Could you check a few things on this model? Use its own coordinates, in mm. A direction names the side the tool comes from. Coordinates: 2 decimals unless noted, no trailing zeros. Write each loop counter-clockwise with the first axis right and the second up, starting at its lowest first coordinate (ties: lowest second). Pieces come first, ordered by that corner, then holes. Notation, with made-up numbers: (82.25, 55) - (99.25, 55) arc R15 cw to (99.25, 66) - close; hole circle Ø6 at (26, 44.25). An arc over 180 degrees is marked (long way). Answer as a JSON object with one key per item and string values. Group by question number.
1) On a 3-axis mill with a long thin cutter (end or side, diameter ignored), from which of +Z, -Z, +X, -X, +Y, -Y can I reach the whole of each face in a straight line? I mean faces 5 (the flat face through (20.15, 0, 33)), 6 (the flat face through (-26.15, 0, 2)), 7 (the flat face through (20.15, 0, 13)), 8 (the cylindrical face through (-10.9, -0.1, 40)), 9 (the flat face through (-24, 0, 29.15)). Say none if no direction works.
2) Will these pins go through, and if not, where does the flat tip stop? pin 1 Ø2.5 at (x, y) = (23.5, 0) entering from -Z; pin 2 Ø6 at (x, y) = (1.5, 4) entering from +Z; pin 3 Ø4 at (x, z) = (-23.5, 1.5) entering from +Y; pin 4 Ø4 at (x, z) = (-21.5, 1.5) entering from -Y.
3) Please list where these lines run through material, in increasing order: line 1 along Y through (x, z) = (24.5, 28.65); line 2 along Z through (x, y) = (-7.9, 3.75); line 3 along X through (y, z) = (3.75, 31.5).
4) We'd pull the mould along Z, two halves only. Please class faces 1 (the cylindrical face through (-6.514, -0.139, 13.425)), 2 (the flat face through (-23, 2.5, 2)), 3 (the flat face through (24, 0, 26.6)), 4 (the flat face through (-24, 0, 26.6)): released by +Z, released by -Z, zero draft, split by the parting line, or undercut.
5) If we section it at C-C (x = 24.5): Write out the boundary of the cut face in (y, z), plus the area to 3 significant figures.
6) If we section it at B-B (x = -24.5): Write out the boundary of the cut face in (y, z).
7) If we section it at A-A (y = -5): Write out the boundary of the cut face in (x, z).
8) If we section it at D-D (y = 0): Write out the boundary of the cut face in (x, z), plus the area to 3 significant figures.
Autodesk Inventor part; units mm, degrees
ref_plane "YZ Plane" through (0, 0, 0) normal (1, 0, 0) x (0, 1, 0)
ref_plane "XZ Plane" through (0, 0, 0) normal (0, 1, 0) x (-1, 0, 0)
ref_plane "XY Plane" through (0, 0, 0) normal (0, 0, 1) x (1, 0, 0)
sketch "Sketch1" plane through (0, 0, 0) normal (0, 0, 1) x (1, 0, 0)
  line L0 (-28.21, 0) -> (28.21, 0)
  line L1 (0, -13.86) -> (0, 13.86)
  line L2 (-20.15, 9.9) -> (20.15, 9.9)
  line L3 (20.15, 9.9) -> (20.15, -9.9)
  line L4 (20.15, -9.9) -> (-20.15, -9.9)
  line L5 (-20.15, -9.9) -> (-20.15, 9.9)
  point P0 (0, 0)
  dimension "d0" = 19.8
  dimension "d1" = 9.9
  dimension "d2" = 40.3
  dimension "d3" = 20.15
extrude "Extrusion1" add sketch "Sketch1" along normal blind 26.6
sketch "Sketch2" plane through (0, 0, 26.6) normal (0, 0, 1) x (1, 0, 0)
  line L0 (-27.75, 9.9) -> (27.75, 9.9)
  line L1 (27.75, 9.9) -> (27.75, -9.9)
  line L2 (27.75, -9.9) -> (-27.75, -9.9)
  line L3 (-27.75, -9.9) -> (-27.75, 9.9)
  line L4 (-38.85, 0) -> (38.85, 0)
  line L5 (0, -13.86) -> (0, 13.86)
  point P0 (0, 0)
  dimension "d6" = 55.5
  dimension "d7" = 19.8
  dimension "d8" = 27.75
  dimension "d9" = 9.9
extrude "Extrusion2" add sketch "Sketch2" along normal blind 2.55
sketch "Sketch3" plane through (0, 0, 29.15) normal (0, 0, 1) x (1, 0, 0)
  line L0 (-27.75, 9.9) -> (27.75, 9.9)
  circle A0 centre (-24.5, 5) radius 2.5
  circle A1 centre (-24.5, -5) radius 2.5
  circle A2 centre (24.5, 5) radius 2.5
  circle A3 centre (24.5, -5) radius 2.5
  point P0 (-27.75, -9.9)
  point P1 (0, 0)
  dimension "d12" = 5
  dimension "d13" = 5
  dimension "d14" = 5
  dimension "d15" = 5
  dimension "d16" = 10
  dimension "d17" = 10
  dimension "d18" = 4.9
  dimension "d19" = 19.8
  dimension "d20" = 4.9
  dimension "d21" = 49
  dimension "d22" = 24.5
extrude "Extrusion3" cut sketch "Sketch3" against normal blind 2.55
sketch "Sketch4" plane through (0, 0, 29.15) normal (0, 0, 1) x (1, 0, 0)
  line L0 (-27.75, 9.9) -> (27.75, 9.9)
  line L1 (27.75, -9.9) -> (-27.75, -9.9)
  line L2 (-20.15, -9.9) -> (-20.15, 9.9)
  line L3 (20.15, 9.9) -> (20.15, -9.9)
  point P0 (0, 0)
extrude "Extrusion4" add sketch "Sketch4" along normal blind 7
sketch "Sketch5" plane through (0, 0, 36.15) normal (0, 0, 1) x (1, 0, 0)
  circle A0 centre (-7.9, 0) radius 3
  line L0 (-27.75, -9.9) -> (-27.75, 9.9)
  point P0 (0, 0)
  dimension "d27" = 6
  dimension "d28" = 19.85
extrude "Extrusion5" add sketch "Sketch5" along normal blind 7.85
sketch "Sketch6" plane through (0, 0, 0) normal (0, 0, -1) x (-1, 0, 0)
  line L0 (20.15, -9.9) -> (20.15, 9.9)
  line L1 (20.15, 2.5) -> (26.15, 2.5)
  line L2 (26.15, 2.5) -> (26.15, -2.5)
  line L3 (26.15, -2.5) -> (20.15, -2.5)
  line L4 (20.15, -2.5) -> (20.15, 2.5)
  point P0 (0, 0)
  dimension "d31" = 6
  dimension "d32" = 2.5
  dimension "d33" = 5
extrude "Extrusion6" add sketch "Sketch6" against normal blind 5
sketch "Sketch7" plane through (-20.15, -9.9, 0) normal (0, -1, 0) x (1, 0, 0)
  line L0 (40.3, 0) -> (0, 0)
  line L1 (9.25, 44) -> (15.25, 44)
  line L2 (9.25, 36.15) -> (9.25, 44)
  line L3 (15.25, 36.15) -> (15.25, 44)
  circle A0 centre (12.25, 14) radius 1.5
  point P0 (20.15, 0)
  dimension "d36" = 3
  dimension "d37" = 30
extrude "Extrusion7" cut sketch "Sketch7" against normal through all
equation "\"d1\" = 0.5 * d0"
equation "\"d3\" = 0.5 * d2"
equation "\"d8\" = 0.5 * d6"
equation "\"d9\" = 0.5 * d7"
equation "\"d20\" = d18"
properties part number "ServoFutabaS3003_UpperArm"
Here are the results:
{
 "1": {"face 5": "+Z, +X, +Y, -Y", "face 6": "-Z, -X, +Y, -Y", "face 7": "-Z, +X, +Y, -Y", "face 8": "+Z", "face 9": "+Z, -X, +Y, -Y"},
 "2": {"pin 1": "stops at z = 26.6", "pin 2": "stops at z = 36.15", "pin 3": "stops at y = 2.5", "pin 4": "stops at y = -9.9"},
 "3": {"line 1": "y = -9.9 to -7.5, -2.5 to 2.5, 7.5 to 9.9", "line 2": "z = 0 to 12.5, 15.5 to 36.15", "line 3": "x = -20.15 to 20.15"},
 "4": {"face 1": "undercut", "face 2": "zero draft", "face 3": "released by -Z", "face 4": "undercut"},
 "5": {"outline": "(-9.9, 26.6) - (-7.5, 26.6) - (-7.5, 29.15) - (-9.9, 29.15) - close; (-2.5, 26.6) - (2.5, 26.6) - (2.5, 29.15) - (-2.5, 29.15) - close; (7.5, 26.6) - (9.9, 26.6) - (9.9, 29.15) - (7.5, 29.15) - close", "area": "25.0 mm²"},
 "6": {"outline": "(-9.9, 26.6) - (-7.5, 26.6) - (-7.5, 29.15) - (-9.9, 29.15) - close; (-2.5, 0) - (2.5, 0) - (2.5, 5) - (-2.5, 5) - close; (-2.5, 26.6) - (2.5, 26.6) - (2.5, 29.15) - (-2.5, 29.15) - close; (7.5, 26.6) - (9.9, 26.6) - (9.9, 29.15) - (7.5, 29.15) - close"},
 "7": {"outline": "(-27.75, 26.6) - (-27, 26.6) - (-27, 29.15) - (-27.75, 29.15) - close; (-22, 26.6) - (-20.15, 26.6) - (-20.15, 0) - (20.15, 0) - (20.15, 26.6) - (22, 26.6) - (22, 29.15) - (20.15, 29.15) - (20.15, 36.15) - (-20.15, 36.15) - (-20.15, 29.15) - (-22, 29.15) - close; (27, 26.6) - (27.75, 26.6) - (27.75, 29.15) - (27, 29.15) - close; hole circle Ø3 at (-7.9, 14)"},
 "8": {"outline": "(-27.75, 26.6) - (-20.15, 26.6) - (-20.15, 5) - (-26.15, 5) - (-26.15, 0) - (20.15, 0) - (20.15, 26.6) - (27.75, 26.6) - (27.75, 29.15) - (20.15, 29.15) - (20.15, 36.15) - (-4.9, 36.15) - (-4.9, 44) - (-10.9, 44) - (-10.9, 36.15) - (-20.15, 36.15) - (-20.15, 29.15) - (-27.75, 29.15) - close; hole circle Ø3 at (-7.9, 14)", "area": "1,570 mm²"}
}
